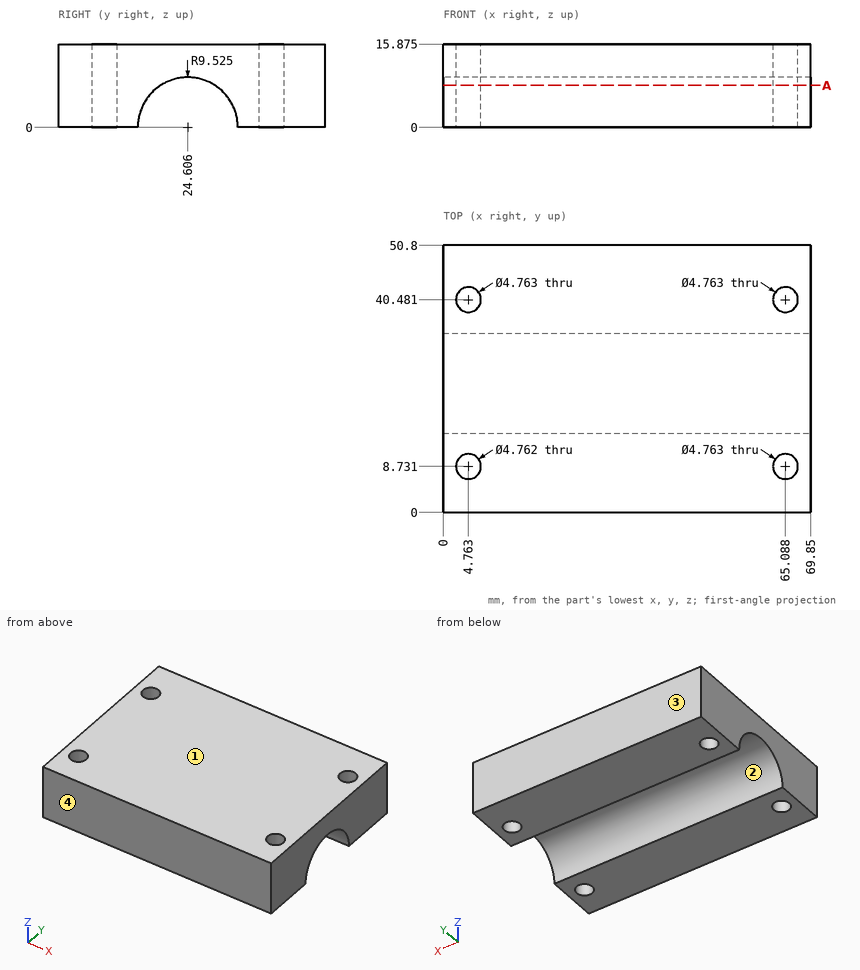
The drawing under review shows one solid part. Ordinate dimensions are in mm from its lowest x, y, z. Coordinates: 2 decimals unless noted, no trailing zeros. Answer as CSV lines item,"result".
Q1. Draft analysis for pull direction Y (two halves, no side actions). For the marked faces 1, 2, 3 and 4, state which applies: released by +Y, released by -Y, zero draft, split by the parting line, or undercut.
Model answer:
face 1,"zero draft"
face 2,"undercut"
face 3,"released by +Y"
face 4,"released by -Y"
Q2. Clearance check with flat-ended pins moving along their axes: pin 1 Ø5 at (x, y) = (37.5, 8.5) entering from -Z; pin 2 Ø4 at (x, y) = (4.76, 40.48) entering from -Z. State where each tip first meets the part, or that it passes through.
Model answer:
pin 1,"stops at z = 0"
pin 2,"passes through"
Q3. We need section A-A (z = 8). Count the separate pieces of the cut face and the enclosed holes in it.
Model answer:
separate pieces,"2"
enclosed holes,"4"
Q4. Wall thickness on line 1 along X through (y, z) = (39.5, 8); line 2 along X through (y, z) = (41, 2.75); line 3 along Y through (x, z) = (38.5, 4): over which ranges is each line inside the solid? List them lowest first. Write a range as [from, to].
Model answer:
line 1,"x = [0, 2.59], [6.93, 62.92], [67.26, 69.85]"
line 2,"x = [0, 2.44], [7.09, 62.76], [67.41, 69.85]"
line 3,"y = [0, 15.96], [33.25, 50.8]"
